Part print with two shaded views. Sizes in mm from the minimum x, y, z corner. Give positions to 0.01 mm unless a question says otherwise; leave off trailing zeros. Write each loop counter-clockwise with the first axis right and the second up, starting at its lowest first coordinate (ties: lowest second). Pieces come first, ordered by that corner, then holes.
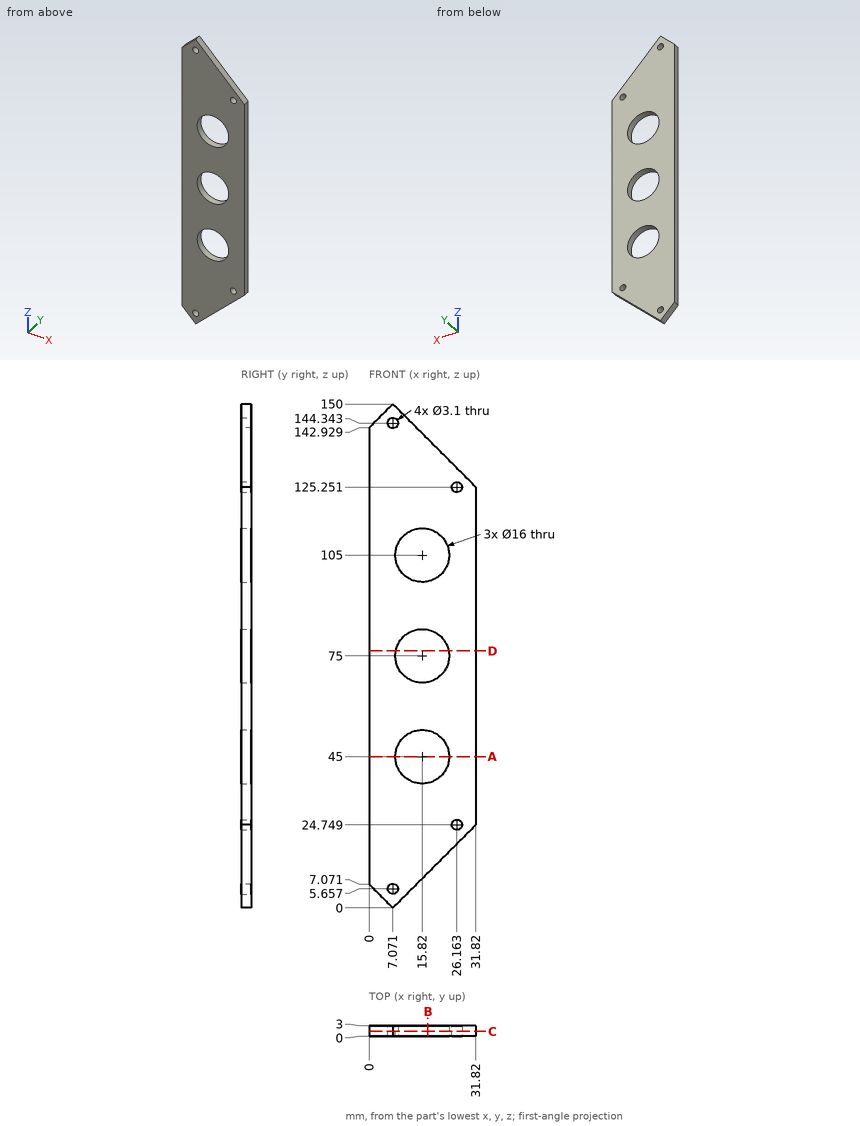
1) Saw through at A-A (z = 45). Write the cut outline in (x, y).
Check result:
outline: (0, 0) - (7.82, 0) - (7.82, 3) - (0, 3) - close; (23.82, 0) - (31.82, 0) - (31.82, 3) - (23.82, 3) - close
2) Saw through at D-D (z = 76.5). Write the cut outline in (x, y).
Check result:
outline: (0, 0) - (7.96, 0) - (7.96, 3) - (0, 3) - close; (23.68, 0) - (31.82, 0) - (31.82, 3) - (23.68, 3) - close
3) Flat gauge pins, fed straight in: P1, Ø2.5, axis at x = 26.16, z = 24.75, coming from the +Y side; P2, Ø1.5, axis at x = 26.5, y = 0.5, coming from the +Z side. Where does each tip first touch, or does it go through?
Check result:
P1: passes through
P2: stops at z = 131.32
4) Saw through at C-C (y = 1.35). Write the cut outline in (x, z).
Check result:
outline: (0, 7.07) - (7.07, 0) - (31.82, 24.75) - (31.82, 125.25) - (7.07, 150) - (0, 142.93) - close; hole circle Ø3.1 at (7.07, 5.66); hole circle Ø3.1 at (7.07, 144.34); hole circle Ø16 at (15.82, 45); hole circle Ø16 at (15.82, 75); hole circle Ø16 at (15.82, 105); hole circle Ø3.1 at (26.16, 24.75); hole circle Ø3.1 at (26.16, 125.25)
5) Saw through at B-B (x = 17.5). Write the cut outline in (y, z), and give its area (3 significant figures).
Check result:
outline: (0, 10.43) - (3, 10.43) - (3, 37.18) - (0, 37.18) - close; (0, 52.82) - (3, 52.82) - (3, 67.18) - (0, 67.18) - close; (0, 82.82) - (3, 82.82) - (3, 97.18) - (0, 97.18) - close; (0, 112.82) - (3, 112.82) - (3, 139.57) - (0, 139.57) - close
area: 247 mm2
6) Drill centre lines: L1, parallel to X at y = 2.25, z = 75; L2, parallel to Z at x = 17, y = 2.75; L3, parallel to Z at x = 6, y = 2.35 (1 decimal). Where is each one in solid material? Low to high.
Check result:
L1: x = 0 to 7.82, 23.82 to 31.82
L2: z = 9.93 to 37.09, 52.91 to 67.09, 82.91 to 97.09, 112.91 to 140.07
L3: z = 1.1 to 4.5, 6.8 to 143.2, 145.5 to 148.9
